Geometry: final body of the model. Coordinates: model frame, mm. Face numbers are marked on the shaded views. A direction names the side the tool comes from. Give positions to 0.01 mm unless a question says otherwise; leave off trailing zeros. Write each loop counter-clockwise with the first axis right and the second up, starting at its lowest first coordinate (ties: lowest second). Pieces come first, ordered by that corner, then holes. Notation, with made-up numbers: (8.5, 21.5) -> (40.5, 21.5) arc R25 ccw to (40.5, 46.5) -> close; hole circle Ø6 at (-10.75, 75.25). An arc over 180 degrees is marked (long way). Answer in a Markdown table with one row per item. Add a question column.
Item 1: Access query for the marked faces 1, 2 and 3. Directions: +Z, -Z, +X, -X, +Y, -Y. A direction counts if a zero-diameter tool reaches every point of the face in a straight line with its end or side. Return the directions, or none.
Item 2: Section query D-D on y = -3. State how many separate pieces and enclosed holes the cut face has, plus the area to 3 significant figures.
Item 3: Section query B-B on x = -7. Output: boundary loops of the cut face in (y, z), plus the area to 3 significant figures.
Item 4: First-contact query: P1, Ø1.6, axis at x = -18, y = -3.5, coming from the -Z side; P2, Ø1.6, axis at x = 16, y = -5, coming from the +Z side; P3, Ø3, axis at x = -18.5, z = -0.5, coming from the -Y side. Flat tips, straight axial feed; report the tip coordinate or a pass-through.
Item 5: Material intervals for probe 1 along X at (y, z) = (-1, -3.5); probe 2 along Z at (x, y) = (-19, -5.25); probe 3 along Y at (x, z) = (-16.5, -1.75), sorted ascending. Write a range as from..to.
Item 6: Section query A-A on z = 0. Output: boundary loops of the cut face in (x, y), plus the area to 3 significant figures.
Item 7: Draft query along Z for the marked faces 4, 5 and 6. Return one class per face: +Z half, -Z half, draft (parallel to the pull), parting line (faces both ways), or undercut.
Item 8: Section query C-C on y = -5.75. Output: boundary loops of the cut face in (x, z), plus the area to 3 significant figures.
```python
from build123d import *

# Parameters (mm, degrees)
EXTRUDE1_DEPTH = 6.5
FILLET1_R      = 1
SHELL2_START   = -6.5
SHELL2_DEPTH   = 5.5
SKETCH2_R      = 15.25
EXTRUDE2_DEPTH = 3.3
EXTRUDE3_DEPTH = 27.626866185
EXTRUDE4_START = -4.3
EXTRUDE4_DEPTH = 4.3
FILLET2_R      = 5


# Read off the part's stored shape, not the designer's step: Shell2
with BuildPart() as part:
    # Sketch1 → Extrude1 (new body)
    with BuildSketch(Plane(origin=(0, 0, 0), x_dir=(1, 0, 0), z_dir=(0, 1, 0))):
        with BuildLine():
            Line((-21.5, 4.25), (-14.371064679, 4.25))
            ThreePointArc((-14.371064679, 4.25), (-13.797975355, 4.430507091), (-13.431779406, 4.906862745))
            ThreePointArc((-13.431779406, 4.906862745), (0, 14.3), (13.431779406, 4.906862745))
            ThreePointArc((13.431779406, 4.906862745), (13.797975355, 4.430507091), (14.371064679, 4.25))
            Line((14.371064679, 4.25), (21.5, 4.25))
            Line((21.5, 4.25), (21.5, -4.25))
            Line((21.5, -4.25), (14.371064679, -4.25))
            ThreePointArc((14.371064679, -4.25), (13.797975355, -4.430507091), (13.431779406, -4.906862745))
            ThreePointArc((13.431779406, -4.906862745), (0, -14.3), (-13.431779406, -4.906862745))
            ThreePointArc((-13.431779406, -4.906862745), (-13.797975355, -4.430507091), (-14.371064679, -4.25))
            Line((-14.371064679, -4.25), (-21.5, -4.25))
            Line((-21.5, -4.25), (-21.5, 4.25))
        make_face()
    extrude(amount=-EXTRUDE1_DEPTH)

    # Fillet1
    fillet1_edges = [part.edges().sort_by_distance(p)[0] for p in [
        (-17.935532339, 0, -4.25),
        (-13.797975355, 0, -4.430507091),
        (0, 0, -14.3),
        (13.797975355, 0, -4.430507091),
        (17.935532339, 0, -4.25),
        (17.935532339, 0, 4.25),
        (13.797975355, 0, 4.430507091),
        (0, 0, 14.3),
        (-13.797975355, 0, 4.430507091),
        (-17.935532339, 0, 4.25),
    ]]
    fillet(fillet1_edges, radius=FILLET1_R)

    # Shell2 outline → Shell2 (cut)
    with BuildSketch(Plane(origin=(0, 0, 0), x_dir=(1, 0, 0), z_dir=(0, 1, 0)).offset(SHELL2_START)):
        with BuildLine():
            ThreePointArc((-12.492494132, 4.56372549), (-13.224886032, 3.611014183), (-14.371064679, 3.25))
            Line((-14.371064679, 3.25), (-21.5, 3.25))
            Line((-21.5, 3.25), (-21.5, -3.25))
            Line((-21.5, -3.25), (-14.371064679, -3.25))
            ThreePointArc((-14.371064679, -3.25), (-13.224886032, -3.611014183), (-12.492494132, -4.56372549))
            ThreePointArc((-12.492494132, -4.56372549), (0, -13.3), (12.492494132, -4.56372549))
            ThreePointArc((12.492494132, -4.56372549), (13.224886032, -3.611014183), (14.371064679, -3.25))
            Line((14.371064679, -3.25), (21.5, -3.25))
            Line((21.5, -3.25), (21.5, 3.25))
            Line((21.5, 3.25), (14.371064679, 3.25))
            ThreePointArc((14.371064679, 3.25), (13.224886032, 3.611014183), (12.492494132, 4.56372549))
            ThreePointArc((12.492494132, 4.56372549), (0, 13.3), (-12.492494132, 4.56372549))
        make_face()
    extrude(amount=SHELL2_DEPTH, mode=Mode.SUBTRACT)

    # Sketch2 → Extrude2 (cut)
    with BuildSketch(Plane.XZ.offset(1)):
        Circle(SKETCH2_R)
    extrude(amount=EXTRUDE2_DEPTH, mode=Mode.SUBTRACT)

    # Sketch4 → Extrude3 (cut, through all)
    with BuildSketch(Plane(origin=(0, 0, 0), x_dir=(1, 0, 0), z_dir=(0, 1, 0))):
        with BuildLine():
            Line((18, 1.761490195), (22, 1.761490195))
            Line((22, 1.761490195), (22, -1.761490195))
            Line((22, -1.761490195), (18, -1.761490195))
            ThreePointArc((18, -1.761490195), (16.238509805, 0), (18, 1.761490195))
        make_face()
        with BuildLine():
            Line((-18, -1.761490195), (-22, -1.761490195))
            Line((-22, -1.761490195), (-22, 1.761490195))
            Line((-22, 1.761490195), (-18, 1.761490195))
            ThreePointArc((-18, 1.761490195), (-16.238509805, 0), (-18, -1.761490195))
        make_face()
    extrude(amount=-EXTRUDE3_DEPTH, mode=Mode.SUBTRACT)

    # Sketch5 → Extrude4 (cut)
    with BuildSketch(Plane(origin=(0, 0, 0), x_dir=(1, 0, 0), z_dir=(0, 1, 0)).offset(EXTRUDE4_START)):
        with BuildLine():
            Line((15, -15), (-15, -15))
            Line((-15, -15), (-15, -3.233227979))
            ThreePointArc((-15, -3.233227979), (-13.629894061, 0), (-15, 3.233227979))
            Line((-15, 3.233227979), (-15, 15))
            Line((-15, 15), (15, 15))
            Line((15, 15), (15, 3.354101966))
            ThreePointArc((15, 3.354101966), (13.5, 0), (15, -3.354101966))
            Line((15, -3.354101966), (15, -15))
        make_face()
    extrude(amount=EXTRUDE4_DEPTH, mode=Mode.SUBTRACT)

    # Fillet2
    fillet2_edges = [part.edges().sort_by_distance(p)[0] for p in [
        (21.5, -6.5, 3.75),
        (-21.5, -6.5, -3.75),
        (-21.5, -6.5, 3.75),
        (21.5, -6.5, -3.75),
    ]]
    fillet(fillet2_edges, radius=FILLET2_R)


solid = part.part
```
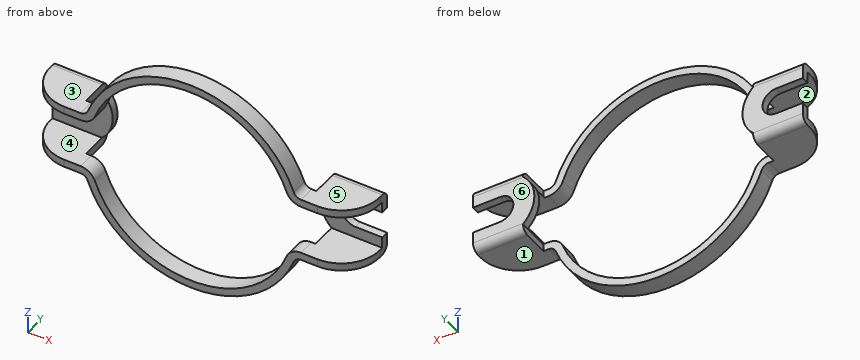
Findings below:
| question | item | result |
|---|---|---|
| 1 | face 1 | -Z, +X, +Y, -Y |
| 1 | face 2 | +X, -X, -Y |
| 1 | face 3 | +Z, -X, +Y, -Y |
| 2 | separate pieces | 4 |
| 2 | enclosed holes | 0 |
| 2 | area | 25.1 mm^2 |
| 3 | outline | (-6.5, -12.47) -> (-4.3, -12.47) -> (-4.3, -11.31) -> (-6.5, -11.31) -> close; (-6.5, 11.31) -> (-4.3, 11.31) -> (-4.3, 12.47) -> (-6.5, 12.47) -> close |
| 3 | area | 5.11 mm^2 |
| 4 | P1 | stops at z = -4.25 |
| 4 | P2 | stops at z = 4.25 |
| 4 | P3 | stops at y = -1 |
| 5 | probe 1 | x = -21.5..-15, 15..21.5 |
| 5 | probe 2 | z = -4.25..-3.25, 3.25..4.25 |
| 5 | probe 3 | y = -1..0 |
| 6 | outline | (-16.24, -1) -> (-13.63, -1) -> (-13.63, 0) -> (-16.24, 0) -> close; (13.5, -1) -> (16.24, -1) -> (16.24, 0) -> (13.5, 0) -> close |
| 6 | area | 5.35 mm^2 |
| 7 | face 4 | undercut |
| 7 | face 5 | +Z half |
| 7 | face 6 | draft |
| 8 | outline | (-19.13, -4.25) -> (-14.37, -4.25) arc R1 cw to (-13.43, -4.91) arc R14.3 ccw to (13.43, -4.91) arc R1 cw to (14.37, -4.25) -> (19.13, -4.25) -> (19.13, -3.25) -> (14.37, -3.25) arc R2 ccw to (12.49, -4.56) arc R13.3 cw to (-12.49, -4.56) arc R2 ccw to (-14.37, -3.25) -> (-19.13, -3.25) -> close; (-19.13, 3.25) -> (-14.37, 3.25) arc R2 ccw to (-12.49, 4.56) arc R13.3 cw to (12.49, 4.56) arc R2 ccw to (14.37, 3.25) -> (19.13, 3.25) -> (19.13, 4.25) -> (14.37, 4.25) arc R1 cw to (13.43, 4.91) arc R14.3 ccw to (-13.43, 4.91) arc R1 cw to (-14.37, 4.25) -> (-19.13, 4.25) -> close |
| 8 | area | 93.7 mm^2 |
